```python
from build123d import *

# Parameters (mm, degrees)
SKETCH1_W              = 76.2
SKETCH1_H              = 134.62
BOSS_EXTRUDE1_DEPTH    = 6.35
SKETCH2_R              = 14.2875
CUT_EXTRUDE1_DEPTH     = 155.820240602
SKETCH3_R              = 3.571875
CUT_EXTRUDE2_DEPTH     = 155.820240602
CHAMFER1_SIZE          = 15.24
F_10_32_TAPPED_HOLE1_D = 4.0386


with BuildPart() as part:
    # Sketch1 → Boss-Extrude1 (new body)
    with BuildSketch(Plane.XY):
        with Locations((38.1, -67.31)):
            Rectangle(SKETCH1_W, SKETCH1_H)
    extrude(amount=BOSS_EXTRUDE1_DEPTH)

    # Sketch2 → Cut-Extrude1 (cut, through all)
    with BuildSketch(Plane.XY.offset(6.35)):
        with Locations((38.1, -41.91)):
            Circle(SKETCH2_R)
    extrude(amount=-CUT_EXTRUDE1_DEPTH, mode=Mode.SUBTRACT)

    # Sketch3 → Cut-Extrude2 (cut, through all)
    with BuildSketch(Plane.XY.offset(6.35)):
        with Locations((12.7, -121.92)):
            Circle(SKETCH3_R)
        with Locations((63.5, -121.92)):
            Circle(SKETCH3_R)
        with Locations((12.7, -96.52)):
            Circle(SKETCH3_R)
        with Locations((63.5, -96.52)):
            Circle(SKETCH3_R)
    extrude(amount=-CUT_EXTRUDE2_DEPTH, mode=Mode.SUBTRACT)

    # Chamfer1
    chamfer1_edges = [part.edges().sort_by_distance(p)[0] for p in [
        (0, 0, 3.175),
        (76.2, 0, 3.175),
    ]]
    chamfer(chamfer1_edges, length=CHAMFER1_SIZE)

    # #10-32 Tapped Hole1 (through all)
    with Locations(Plane.XY.offset(6.35)):
        with Locations((38.1, -22.86)):
            Hole(F_10_32_TAPPED_HOLE1_D / 2)


solid = part.part
```
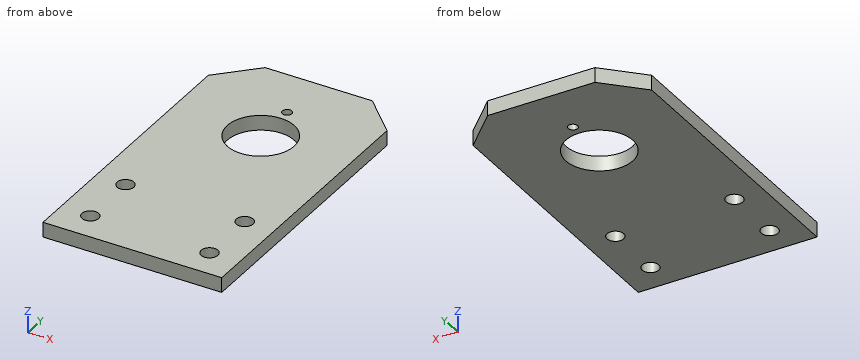
Design review of the part built by this model. Coordinates are the model's own, in mm. Give positions to 0.01 mm unless a question says otherwise; leave off trailing zeros. Write each loop counter-clockwise with the first axis right and the second up, starting at its lowest first coordinate (ties: lowest second). Pieces come first, ordered by that corner, then holes. Notation, with made-up numbers: (35.5, -12.75) - (72.5, -12.75) arc R9 ccw to (72.5, -0.75) - close; hole circle Ø2 at (-38, 54). An arc over 180 degrees is marked (long way). Return JSON: item names as keys, results as strings. Group by question number.
(1) We need section C-C, the plane x = 12.7. Give the boundary of the cut face in (y, z), then the cut area to 3 significant figures.
(2) To check wall thickness, follow probe 1 along Y at (x, z) = (38.1, 2.75); probe 2 along X at (y, z) = (-41, 5.25); probe 3 along X at (y, z) = (-124, 3). State the ranges of each line that lie inside material, in increasing order.
(3) We need section B-B, the plane z = 2.5. Give the boundary of the cut face in (x, y) (1 decimal), then the cut area to 3 significant figures.
(4) We need section D-D, the plane y = -121.92. Give the boundary of the cut face in (x, z), then the cut area to 3 significant figures.
(5) We need section A-A, the plane y = -22.86. Give the boundary of the cut face in (x, z).
Reported:
{
 "1": {"outline": "(-134.62, 0) - (-125.49, 0) - (-125.49, 6.35) - (-134.62, 6.35) - close; (-118.35, 0) - (-100.09, 0) - (-100.09, 6.35) - (-118.35, 6.35) - close; (-92.95, 0) - (-2.54, 0) - (-2.54, 6.35) - (-92.95, 6.35) - close", "area": "748 mm2"},
 "2": {"probe 1": "y = -134.62 to -56.2, -27.62 to -24.88, -20.84 to 0", "probe 2": "x = 0 to 23.84, 52.36 to 76.2", "probe 3": "x = 0 to 9.8, 15.6 to 60.6, 66.4 to 76.2"},
 "3": {"outline": "(0, -134.6) - (76.2, -134.6) - (76.2, -15.2) - (61, 0) - (15.2, 0) - (0, -15.2) - close; hole circle Ø7.1 at (12.7, -121.9); hole circle Ø7.1 at (12.7, -96.5); hole circle Ø28.6 at (38.1, -41.9); hole circle Ø4 at (38.1, -22.9); hole circle Ø7.1 at (63.5, -121.9); hole circle Ø7.1 at (63.5, -96.5)", "area": "9,210 mm2"},
 "4": {"outline": "(0, 0) - (9.13, 0) - (9.13, 6.35) - (0, 6.35) - close; (16.27, 0) - (59.93, 0) - (59.93, 6.35) - (16.27, 6.35) - close; (67.07, 0) - (76.2, 0) - (76.2, 6.35) - (67.07, 6.35) - close", "area": "393 mm2"},
 "5": {"outline": "(0, 0) - (36.08, 0) - (36.08, 6.35) - (0, 6.35) - close; (40.12, 0) - (76.2, 0) - (76.2, 6.35) - (40.12, 6.35) - close"}
}
